Job drawing, mm, ordinate dimensions from the low corner. One solid piece. A direction names the side the tool comes from. Coordinates: 2 decimals unless noted, no trailing zeros. Order: outer loops, then holes, each group sorted by start corner. A loop starts at its lowest first (then second) coordinate and runs counter-clockwise, first axis right, second up. Notation, with made-up numbers: (45, 69.25) - (76, 69.25) arc R20 ccw to (76, 82.25) - close; hole circle Ø1 at (12, -34.5). An arc over 180 degrees is marked (long way). Use one line per item in the form item = value.
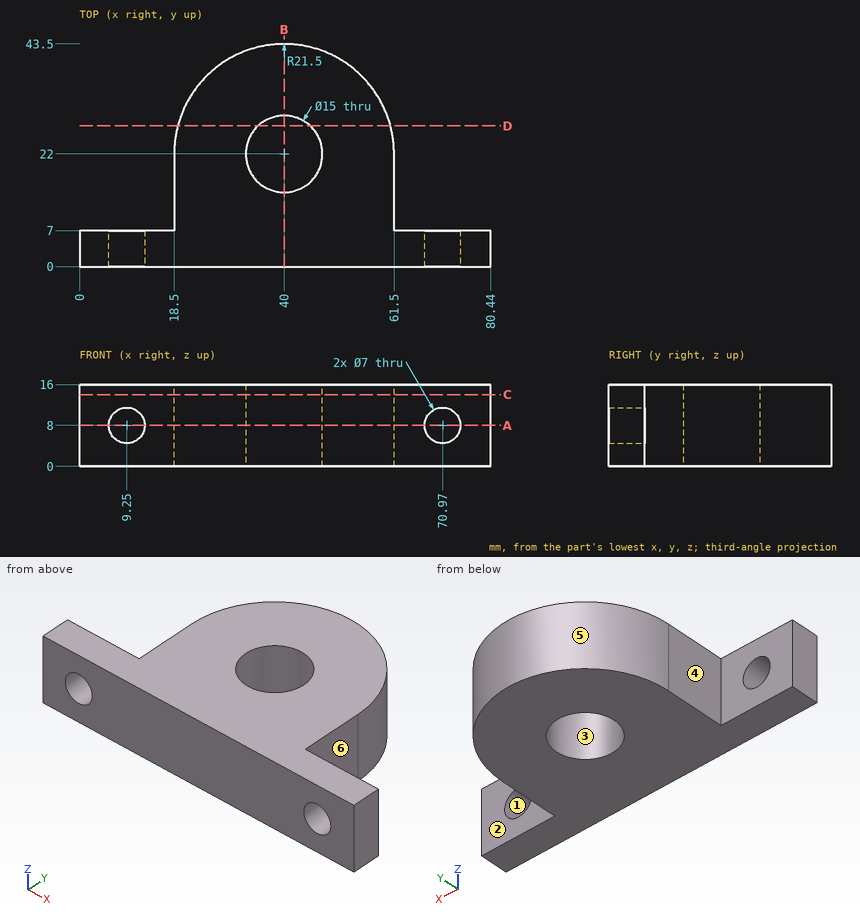
Item 1: Cut at B-B, the plane x = 40. Write the cut outline in (y, z), plus the area to 3 significant figures.
Derived:
outline = (0, 0) - (14.5, 0) - (14.5, 16) - (0, 16) - close; (29.5, 0) - (43.5, 0) - (43.5, 16) - (29.5, 16) - close
area = 456 mm²
Item 2: Drop flat-ended pins along their axis: pin 1 (4 mm diameter, centred on x = 9.25, z = 8, fed in from +Y); pin 2 (8 mm diameter, centred on x = 21.5, z = 9, fed in from -Y); pin 3 (6 mm diameter, centred on x = 43, z = 3.5, fed in from +Y); pin 4 (4.5 mm diameter, centred on y = 16.5, z = 8.5, fed in from +X). Give the stop position or say it passes through.
Derived:
pin_1 = through
pin_2 = 0
pin_3 = 43.5
pin_4 = 61.5
Item 3: Cut at C-C, the plane z = 14. Write the cut outline in (x, y).
Derived:
outline = (0, 0) - (80.44, 0) - (80.44, 7) - (61.5, 7) - (61.5, 22) arc R21.5 ccw to (18.5, 22) - (18.5, 7) - (0, 7) - close; hole circle Ø15 at (40, 22)
Item 4: Cut at D-D, the plane y = 27.5. Write the cut outline in (x, z), plus the area to 3 significant figures.
Derived:
outline = (19.22, 0) - (34.9, 0) - (34.9, 16) - (19.22, 16) - close; (45.1, 0) - (60.78, 0) - (60.78, 16) - (45.1, 16) - close
area = 502 mm²
Item 5: 3-axis set-ups, long thin cutter, end or side, ignore diameter. For the marked faces 4, 5 and 6: which of +Z, -Z, +X, -X, +Y, -Y reach the whole face in a straight line?
Derived:
face_4 = +Z, -Z, -X, +Y
face_5 = +Z, -Z, +Y
face_6 = +Z, -Z, +X, +Y
Item 6: Drill centre lines: line 1 (X direction, y = 5.75, z = 8); line 2 (Y direction, x = 40, z = 3.75); line 3 (Z direction, x = 9, y = 4). Where is each one in solid material? Low to high. Write a range as [from, to].
Derived:
line_1 = [0, 5.75], [12.75, 67.47], [74.47, 80.44]
line_2 = [0, 14.5], [29.5, 43.5]
line_3 = [0, 4.51], [11.49, 16]
Item 7: Cut at A-A, the plane z = 8. Write the cut outline in (x, y).
Derived:
outline = (0, 0) - (5.75, 0) - (5.75, 7) - (0, 7) - close; (12.75, 0) - (67.47, 0) - (67.47, 7) - (61.5, 7) - (61.5, 22) arc R21.5 ccw to (18.5, 22) - (18.5, 7) - (12.75, 7) - close; (74.47, 0) - (80.44, 0) - (80.44, 7) - (74.47, 7) - close; hole circle Ø15 at (40, 22)
Item 8: Two-plate mould, pull along Y, no slides. Class the marked faces 1, 2 and 3: +Y half, -Y half, draft (parallel to the pull), parting line (faces both ways), or undercut.
Derived:
face_1 = draft
face_2 = +Y half
face_3 = undercut
